Input: part model. Units: mm. Frame: model coordinates. Coordinates: 2 decimals unless noted, no trailing zeros. Loops run counter-clockwise (first coordinate to the right, second up) from the corner with the lowest first, then second, coordinate; pieces in that order, holes last. Notation, with made-up numbers: (57.25, -21.5) - (105.25, -21.5) arc R17 ccw to (105.25, 10.5) - close; hole circle Ø6 at (-27.5, 69.25). An arc over 180 degrees is marked (long way). Use a Markdown table: item, result. Add a question column.
1. Section query B-B on z = 7. Return the cut outline in (x, y).
2. Draft query along Z for faces 1 (the face through (-0.175, 0.751, 7.385)), 2 (the face through (0, 0, 15)), 3 (the face through (0, 15, 7)). Return one class per face: released by +Z, released by -Z, zero draft, split by the parting line, or undercut.
3. Section query C-C on x = -1.5. Return the cut outline in (y, z), then the cut area to 3 significant figures.
4. Section query A-A on y = 0. Return the cut outline in (x, z).
5. Ray query, L1, parallel to Y at x = 5.5, z = 5; L2, parallel to Y at x = 3.75, z = 3.5; L3, parallel to Z at x = -2.25, y = 2.25. Return the intervals inside material, ascending. Write a range as [from, to].
```python
from build123d import *

# Parameters (mm, degrees)
SKETCH1_W           = 25
SKETCH1_H           = 30
BOSS_EXTRUDE1_DEPTH = 15
SKETCH2_R           = 2.5
CUT_EXTRUDE1_DEPTH  = 26


with BuildPart() as part:
    # Sketch1 → Boss-Extrude1 (new body)
    with BuildSketch(Plane.XY):
        Rectangle(SKETCH1_W, SKETCH1_H)
    extrude(amount=BOSS_EXTRUDE1_DEPTH)

    # Sketch2 → Cut-Extrude1 (cut)
    with BuildSketch(Plane.ZY.offset(12.5)):
        with Locations((5, 0)):
            Circle(SKETCH2_R)
    extrude(amount=-CUT_EXTRUDE1_DEPTH, mode=Mode.SUBTRACT)


solid = part.part
```
Resolved:
| question | item | result |
|---|---|---|
| 1 | outline | (-12.5, -15) - (12.5, -15) - (12.5, -1.5) - (-12.5, -1.5) - close; (-12.5, 1.5) - (12.5, 1.5) - (12.5, 15) - (-12.5, 15) - close |
| 2 | face 1 | undercut |
| 2 | face 2 | released by +Z |
| 2 | face 3 | zero draft |
| 3 | outline | (-15, 0) - (15, 0) - (15, 15) - (-15, 15) - close; hole circle Ø5 at (0, 5) |
| 3 | area | 430 mm² |
| 4 | outline | (-12.5, 0) - (12.5, 0) - (12.5, 2.5) - (-12.5, 2.5) - close; (-12.5, 7.5) - (12.5, 7.5) - (12.5, 15) - (-12.5, 15) - close |
| 5 | L1 | [-15, -2.5], [2.5, 15] |
| 5 | L2 | [-15, -2], [2, 15] |
| 5 | L3 | [0, 3.91], [6.09, 15] |
